Could you check a few things on this model? Use its own coordinates, in mm. A direction names the side the tool comes from. Give positions to 0.01 mm unless a question says otherwise; leave off trailing zeros. Order: outer loops, then holes, each group sorted by start corner. A loop starts at its lowest first (then second) coordinate and runs counter-clockwise, first axis right, second up. Notation, with made-up numbers: M 46.5,59 L 96.5,59 A15 cw 96.5,70 Z; hole C 74,6.25 d10. An arc over 180 degrees is marked long. Return JSON: item names as keys, results as strings. Group by question number.
```python
from build123d import *

# Parameters (mm, degrees)
BOSS_EXTRUDE1_DEPTH = 5
SKETCH2_R           = 5
BOSS_EXTRUDE2_DEPTH = 1
SKETCH3_R           = 3.555
BOSS_EXTRUDE3_DEPTH = 2.5
SKETCH4_R           = 2.5
CUT_EXTRUDE1_DEPTH  = 9.5
CUT_EXTRUDE2_DEPTH  = 4.5


with BuildPart() as part:
    # Sketch1 → Boss-Extrude1 (new body)
    with BuildSketch(Plane(origin=(0, 0, 0), x_dir=(1, 0, 0), z_dir=(0, 1, 0))):
        Polygon((4.543746619, 0), (2.271873309, 3.935), (-2.271873309, 3.935), (-4.543746619, 0), (-2.271873309, -3.935), (2.271873309, -3.935), align=None)
    extrude(amount=BOSS_EXTRUDE1_DEPTH)

    # Sketch2 → Boss-Extrude2 (add)
    with BuildSketch(Plane(origin=(0, 0, 0), x_dir=(1, 0, 0), z_dir=(0, 1, 0))):
        Circle(SKETCH2_R)
    extrude(amount=-BOSS_EXTRUDE2_DEPTH)

    # Sketch3 → Boss-Extrude3 (add)
    with BuildSketch(Plane.XZ.offset(1)):
        Circle(SKETCH3_R)
    extrude(amount=BOSS_EXTRUDE3_DEPTH)

    # Sketch4 → Cut-Extrude1 (cut, through all)
    with BuildSketch(Plane(origin=(0, 5, 0), x_dir=(1, 0, 0), z_dir=(0, 1, 0))):
        with Locations((0, -0.79)):
            Circle(SKETCH4_R)
    extrude(amount=-CUT_EXTRUDE1_DEPTH, mode=Mode.SUBTRACT)

    # Sketch5 → Cut-Extrude2 (cut, through all)
    with BuildSketch(Plane(origin=(0, 0, 0), x_dir=(1, 0, 0), z_dir=(0, 1, 0))):
        with BuildLine():
            Line((-1.7, -4.702127178), (1.7, -4.702127178))
            ThreePointArc((1.7, -4.702127178), (0, -5), (-1.7, -4.702127178))
        make_face()
    extrude(amount=-CUT_EXTRUDE2_DEPTH, mode=Mode.SUBTRACT)

    # Sketch6 → Cut-Revolve1 (revolve, cut)
    with BuildSketch(Plane.XY):
        Polygon((4.043746619, 5), (4.543746619, 5), (4.543746619, 4.5), align=None)
    revolve(axis=Axis((0, 0, 0), (0, 1, 0)), mode=Mode.SUBTRACT)


solid = part.part
```
1. Imagine slicing it at C-C, the plane z = 2.25. Please give me the cut outline in (x, y).
2. I need wall thicknesses on L1, parallel to Z at x = 0, y = 2 (3 decimals); L2, parallel to Z at x = 0, y = -0.75; L3, parallel to X at y = 0.75, z = 0.79. Which ranges of each line are inside material? Lowest first, please. Write a range as from..to.
3. Which directions (+Z, -Z, +X, -X, +Y, -Y) give clear straight access to the entire face, cutting with the end or side of a thin tool? Please do faces 1 (the flat face through (2.2, -1, 3)), 2 (the flat face through (-3.4, 0, -2.3)), 3 (the flat face through (-3.424, 2.465, 1.94)), 4 (the flat face through (3.424, 2.465, -1.94)).
4. If we mould it in two halves opening along Z, with no side actions, what happens to faces 5 (the cylindrical face through (0.196, -0.493, -4.996)), 6 (the conical face through (2.104, 4.865, -3.611)), 7 (the cylindrical face through (-0.54, 0.81, 3.23)), 8 (the conical face through (2.075, 4.865, 3.628))? For each: pulls with the +Z half, pulls with the -Z half, needs draft (parallel to the pull), parting line crosses it, or undercut.
5. Imagine slicing it at A-A, the plane x = 0. Please give me the cut outline in (y, z) (3 decimals), plus the area to 3 significant figures.
6. For pin 1 (1.4 mm diameter, centred on x = -1, y = 1.5, fed in from -Z) (3 decimals); pin 2 (1 mm diameter, centred on x = 3.5, y = 1.5, fed in from -Z), each with a flat end and sliding along its axis, tell me the tip position at first contact or that it passes through.
7. Imagine slicing it at B-B, the plane y = 0.25. Please give me the cut outline in (x, z) (3 decimals).
Values:
{
 "1": {"outline": "M -4.47,-1 L -2.75,-1 L -2.75,-3.5 L -2.03,-3.5 L -2.03,5 L -3.24,5 L -3.24,0 L -4.47,0 Z; M 2.03,-3.5 L 2.75,-3.5 L 2.75,-1 L 4.47,-1 L 4.47,0 L 3.24,0 L 3.24,5 L 2.03,5 Z"},
 "2": {"L1": "z = -3.935..-1.71, 3.29..3.935", "L2": "z = -5..-1.71, 3.29..4.7", "L3": "x = -4.09..-2.5, 2.5..4.09"},
 "3": {"face 1": "-Y", "face 2": "+Y", "face 3": "+Z, -X, +Y", "face 4": "-Z, +X, +Y"},
 "4": {"face 5": "parting line crosses it", "face 6": "pulls with the -Z half", "face 7": "undercut", "face 8": "pulls with the +Z half"},
 "5": {"outline": "M -3.5,-3.555 L -1,-3.555 L -1,-5 L 0,-5 L 0,-3.935 L 5,-3.935 L 5,-1.71 L -3.5,-1.71 Z; M -3.5,3.29 L 5,3.29 L 5,3.935 L 0,3.935 L 0,4.702 L -1,4.702 L -1,3.555 L -3.5,3.555 Z", "area": "24.3 mm²"},
 "6": {"pin 1": "stops at z = -3.935", "pin 2": "stops at z = -2.67"},
 "7": {"outline": "M -4.544,0 L -2.272,-3.935 L 2.272,-3.935 L 4.544,0 L 2.272,3.935 L -2.272,3.935 Z; hole C 0,0.79 d5"}
}
